Part print with two shaded views. Sizes in mm from the minimum x, y, z corner. Coordinates: 2 decimals unless noted, no trailing zeros. Write each loop counter-clockwise with the first axis right and the second up, starting at its lowest first coordinate (ties: lowest second). Pieces come first, ordered by that corner, then holes. Notation, with made-up numbers: (72, 44) - (103, 44) arc R21 ccw to (103, 54) - close; hole circle Ø8 at (60.5, 44). An arc over 180 degrees is marked (long way). Answer in a Markdown table with one row per item. Add a question column.
Q1. Drill centre lines: line 1 along Y through (x, z) = (25, 1.25); line 2 along Y through (x, z) = (26.5, 3.25); line 3 along X through (y, z) = (113.6, 1.55). Where is each one in solid material? Low to high. Write a range as from..to.
Q2. Pin check, flat tip, straight feed: pin 1 (5 mm diameter, centred on x = 25, y = 39.551, fed in from -Z). Stop position of the tip, or through.
Q3. Band-saw the part on A-A (x = 25). List the corners of the cut face in (y, z).
Q4. Band-saw the part on B-B (y = 113.6). List the corners of the cut face in (x, z), and give its area (3 significant figures).
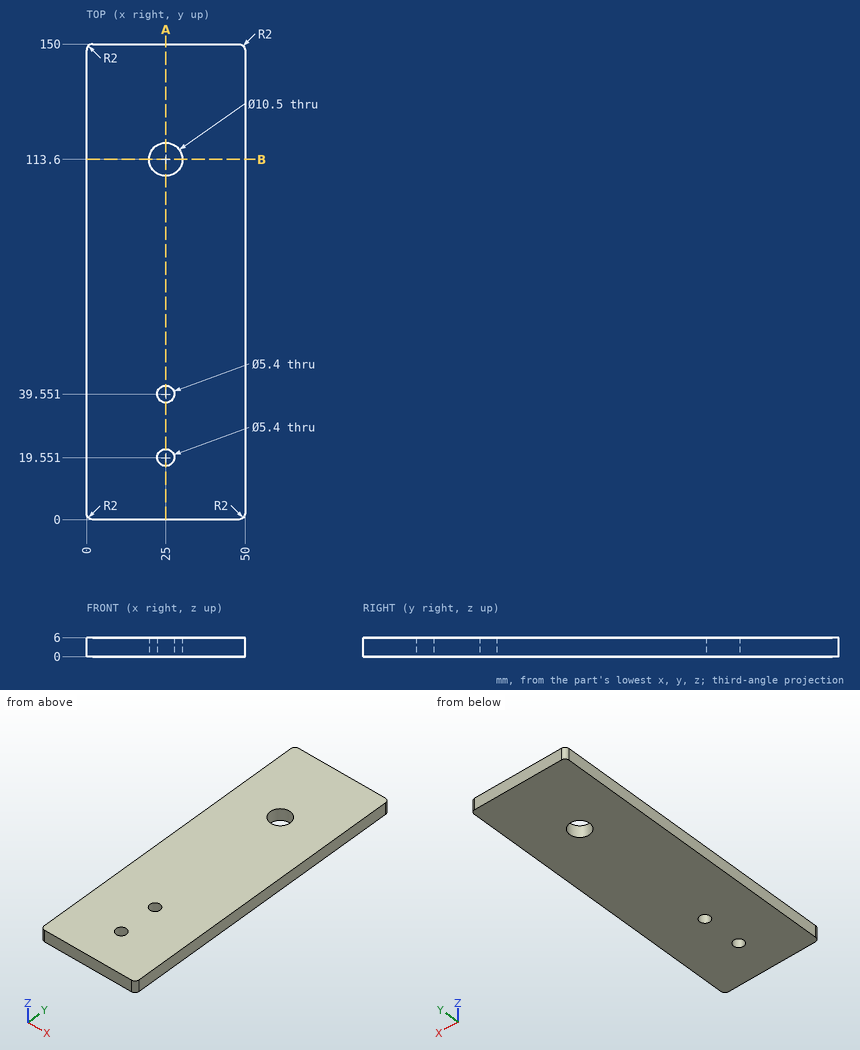
Checked values:
| question | item | result |
|---|---|---|
| 1 | line 1 | y = 0..16.85, 22.25..36.85, 42.25..108.35, 118.85..150 |
| 1 | line 2 | y = 0..17.31, 21.8..37.31, 41.8..108.57, 118.63..150 |
| 1 | line 3 | x = 0..19.75, 30.25..50 |
| 2 | pin 1 | passes through |
| 3 | outline | (0, 0) - (16.85, 0) - (16.85, 6) - (0, 6) - close; (22.25, 0) - (36.85, 0) - (36.85, 6) - (22.25, 6) - close; (42.25, 0) - (108.35, 0) - (108.35, 6) - (42.25, 6) - close; (118.85, 0) - (150, 0) - (150, 6) - (118.85, 6) - close |
| 4 | outline | (0, 0) - (19.75, 0) - (19.75, 6) - (0, 6) - close; (30.25, 0) - (50, 0) - (50, 6) - (30.25, 6) - close |
| 4 | area | 237 mm² |
